```python
from build123d import *

# Parameters (mm, degrees)
SKETCH1_R           = 3.3734375
SKETCH1_R_2         = 6.35
SKETCH1_R_3         = 31.75
BOSS_EXTRUDE1_DEPTH = 6.35
FILLET1_R           = 3.175


with BuildPart() as part:
    # Sketch1 → Boss-Extrude1 (new body)
    with BuildSketch(Plane(origin=(0, 0, 0), x_dir=(0, 0, -1), z_dir=(1, 0, 0))):
        Polygon((0, 0), (546.1, 0), (455.432604376, 181.850662278), (478.163937161, 193.184086731), (387.496541537, 375.034749008), (364.765208752, 363.701324555), (280.156570264, 533.4), (265.943429736, 533.4), (182.751469304, 366.542741153), (194.117135697, 360.876028927), (100.61638396, 173.342533453), (89.250717567, 179.009245679), align=None)
        with Locations((171.45, 19.05)):
            Circle(SKETCH1_R, mode=Mode.SUBTRACT)
        with Locations((374.65, 19.05)):
            Circle(SKETCH1_R, mode=Mode.SUBTRACT)
        with Locations((410.098906564, 272.775993416)):
            Circle(SKETCH1_R_2, mode=Mode.SUBTRACT)
        with Locations((170.098092613, 255.775856737)):
            Circle(SKETCH1_R_2, mode=Mode.SUBTRACT)
        with Locations((171.579254548, 201.821183313)):
            Circle(SKETCH1_R_3, mode=Mode.SUBTRACT)
        with Locations((408.617744629, 218.821319992)):
            Circle(SKETCH1_R_3, mode=Mode.SUBTRACT)
    extrude(amount=BOSS_EXTRUDE1_DEPTH)

    # Fillet1
    fillet1_edges = [part.edges().sort_by_distance(p)[0] for p in [
        (3.175, 179.009245679, -89.250717567),
        (3.175, 173.342533453, -100.61638396),
        (3.175, 360.876028927, -194.117135697),
        (3.175, 366.542741153, -182.751469304),
        (3.175, 533.4, -265.943429736),
        (3.175, 533.4, -280.156570264),
        (3.175, 363.701324555, -364.765208752),
        (3.175, 375.034749008, -387.496541537),
        (3.175, 193.184086731, -478.163937161),
        (3.175, 181.850662278, -455.432604376),
        (3.175, 0, -546.1),
        (3.175, 0, 0),
    ]]
    fillet(fillet1_edges, radius=FILLET1_R)


solid = part.part
```
CAD build for the part. Positions are in the model's coordinates, mm. A direction names the side the tool comes from. Round coordinates to 2 decimals unless told otherwise and drop trailing zeros. Write each loop counter-clockwise with the first axis right and the second up, starting at its lowest first coordinate (ties: lowest second). Pieces come first, ordered by that corner, then holes.
Item 1: Band-saw the part on C-C on y = 312. Write the cut outline in (x, z).
Filled in:
outline: (0, -418.92) - (6.35, -418.92) - (6.35, -169.75) - (0, -169.75) - close
Item 2: Mould opens along Z. For faces 3 (the flat face through (3.13, 91.58, -45.66)), 4 (the cylindrical face through (3.131, 256.055, -163.754)), 5 (the flat face through (6.35, 211, -269)) say: released by +Z, released by -Z, zero draft, split by the parting line, or undercut.
Filled in:
face 3: released by +Z
face 4: undercut
face 5: zero draft
Item 3: Drill centre lines: L1, parallel to Z at x = 3.25, y = 215.5; L2, parallel to Y at x = 3.25, z = -171.45; L3, parallel to Z at x = 4.75, y = 218. Where is each one in solid material? Low to high.
Filled in:
L1: z = -467.04 to -440.19, -377.04 to -200.23, -142.93 to -121.64
L2: y = 0 to 15.68, 22.42 to 170.07, 233.57 to 249.57, 261.98 to 315.41
L3: z = -465.79 to -440.36, -376.88 to -198.9, -144.26 to -122.88
Item 4: Tool access for faces 1 (the flat face through (3.131, 282.876, -433.445)), 2 (the flat face through (3.13, 90.58, -500.94)): list every direction of +Z, -Z, +X, -X, +Y, -Y with a clear straight run to the whole face (end or side of a thin tool).
Filled in:
face 1: -Z, +X, -X, +Y
face 2: -Z, +X, -X
Item 5: Drop a flat-ended pin along its axis: pin 1 Ø1 at (x, y) = (5.5, 73) entering from -Z. Give the stop position or say it passes through.
Filled in:
pin 1: stops at z = -509.95
Item 6: Band-saw the part on A-A on x = 4.5. Give the number of separate pieces and of enclosed holes in the cut face, then the cut area to 3 significant figures.
Filled in:
separate pieces: 1
enclosed holes: 6
area: 145,000 mm2
Item 7: Band-saw the part on B-B on z = -60.5. Write the cut outline in (x, y).
Filled in:
outline: (0, 0) - (6.35, 0) - (6.35, 121.34) - (0, 121.34) - close
